Job drawing, mm, ordinate dimensions from the low corner. One solid piece. Give positions to 0.01 mm unless a question says otherwise; leave off trailing zeros. Write each loop counter-clockwise with the first axis right and the second up, starting at its lowest first coordinate (ties: lowest second). Pieces come first, ordered by that corner, then holes. Notation, with made-up numbers: (7.25, 11) -> (26.25, 11) arc R16 cw to (26.25, 31) -> close; hole circle Ø8 at (64.25, -39.75). An arc over 180 degrees is marked (long way). Put each result on its own line as item: value. Start each with the question number.
Item 1: Slice it at A-A, the plane x = 63.75. List the corners of the cut face in (y, z) (3 decimals), plus the area to 3 significant figures.
Item 2: Drill centre lines: line 1 along Y through (x, z) = (16.25, 1.6); line 2 along Y through (x, z) = (61.5, 5.4); line 3 along Y through (x, z) = (37.5, 2.65). Where is each one in solid material? Low to high.
Item 3: Flat gauge pins, fed straight in: pin 1 Ø5.5 at (x, y) = (63.75, 77) entering from -Z; pin 2 Ø3 at (x, y) = (62.5, 77.5) entering from +Z; pin 3 Ø1.8 at (x, z) = (40, 3) entering from +Y. Where does each tip first touch, or does it go through?
Item 4: Slice it at B-B, the plane y = 77. List the corners of the cut face in (x, z) (3 decimals).
Item 5: Slice it at C-C, the plane z = 1.7. List the corners of the cut face in (x, y).
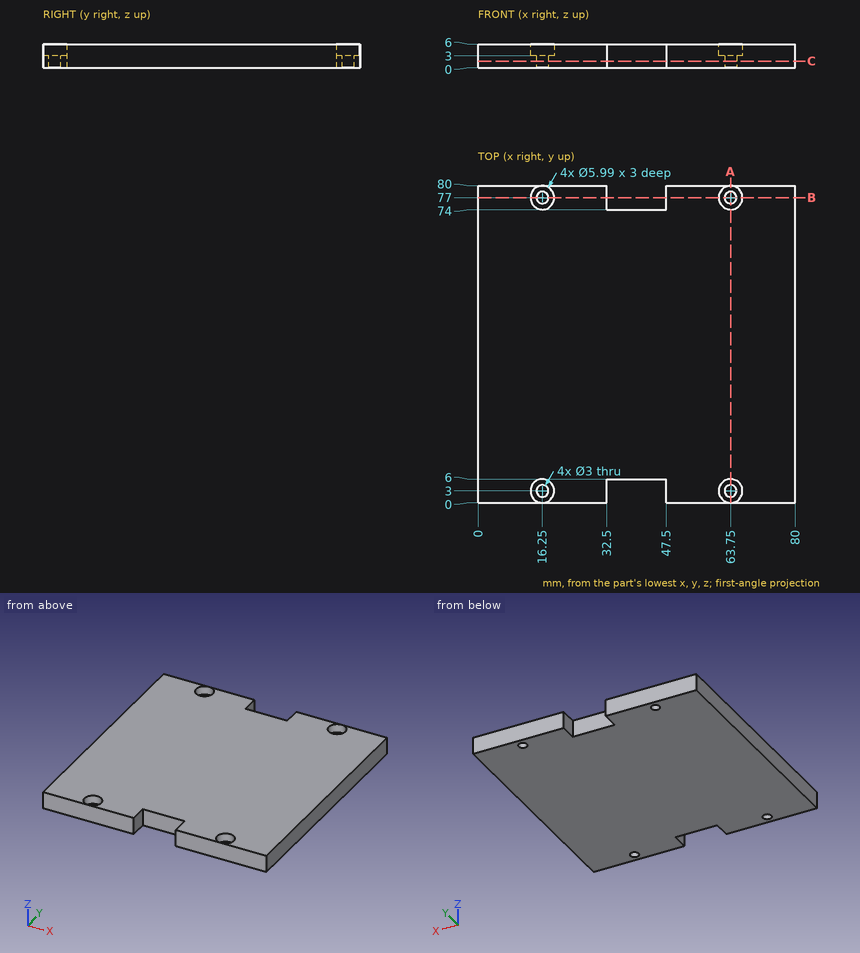
Values follow:
1. outline: (0, 0) -> (1.5, 0) -> (1.5, 3) -> (0.005, 3) -> (0.005, 6) -> (0, 6) -> close; (4.5, 0) -> (75.5, 0) -> (75.5, 3) -> (74.005, 3) -> (74.005, 6) -> (5.995, 6) -> (5.995, 3) -> (4.5, 3) -> close; (78.5, 0) -> (80, 0) -> (80, 6) -> (79.995, 6) -> (79.995, 3) -> (78.5, 3) -> close
1. area: 426 mm2
2. line 1: 0 to 1.5, 4.5 to 75.5, 78.5 to 80
2. line 2: 0 to 1.02, 4.98 to 75.02, 78.98 to 80
2. line 3: 6 to 74
3. pin 1: z = 0
3. pin 2: z = 3
3. pin 3: y = 74
4. outline: (0, 0) -> (14.75, 0) -> (14.75, 3) -> (13.255, 3) -> (13.255, 6) -> (0, 6) -> close; (17.75, 0) -> (32.5, 0) -> (32.5, 6) -> (19.245, 6) -> (19.245, 3) -> (17.75, 3) -> close; (47.5, 0) -> (62.25, 0) -> (62.25, 3) -> (60.755, 3) -> (60.755, 6) -> (47.5, 6) -> close; (65.25, 0) -> (80, 0) -> (80, 6) -> (66.745, 6) -> (66.745, 3) -> (65.25, 3) -> close
5. outline: (0, 0) -> (32.5, 0) -> (32.5, 6) -> (47.5, 6) -> (47.5, 0) -> (80, 0) -> (80, 80) -> (47.5, 80) -> (47.5, 74) -> (32.5, 74) -> (32.5, 80) -> (0, 80) -> close; hole circle Ø3 at (16.25, 3); hole circle Ø3 at (16.25, 77); hole circle Ø3 at (63.75, 3); hole circle Ø3 at (63.75, 77)
